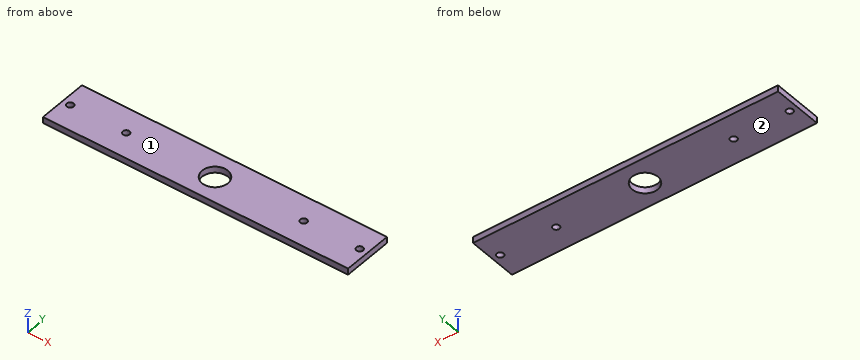
from build123d import *

# Parameters (mm, degrees)
SKETCH1_W               = 311.15
SKETCH1_H               = 50.8
BOSS_EXTRUDE1_DEPTH     = 6.35
F_1_CLEARANCE_HOLE1_D   = 26.19248
F_1_4_CLEARANCE_HOLE1_D = 6.7564


with BuildPart() as part:
    # Sketch1 → Boss-Extrude1 (new body)
    with BuildSketch(Plane.XY):
        Rectangle(SKETCH1_W, SKETCH1_H)
    extrude(amount=BOSS_EXTRUDE1_DEPTH)

    # 1 Clearance Hole1 (through all)
    with Locations(Plane.XY.offset(6.35)):
        with Locations((0, 0)):
            Hole(F_1_CLEARANCE_HOLE1_D / 2)

    # 1/4 Clearance Hole1 (through all)
    with Locations(Plane.XY.offset(6.35)):
        with Locations((-147.6375, 0), (-90.4875, 0)):
            f_1_4_clearance_hole1 = Hole(F_1_4_CLEARANCE_HOLE1_D / 2)

    # Mirror1: 1/4 Clearance Hole1 across plane
    add(f_1_4_clearance_hole1.mirror(Plane(origin=(0, 0, 0), x_dir=(0, 0, 1), z_dir=(1, 0, 0))), mode=Mode.SUBTRACT)


solid = part.part
Geometry: final body of the model. Coordinates: model frame, mm. Face numbers are marked on the shaded views. Round coordinates to 2 decimals unless told otherwise and drop trailing zeros. Order: outer loops, then holes, each group sorted by start corner. A loop starts at its lowest first (then second) coordinate and runs counter-clockwise, first axis right, second up. Notation, with made-up numbers: (3.5, -7.5) -> (48.5, -7.5) arc R8 ccw to (48.5, -0.5) -> close; hole circle Ø11 at (41, 7.25). An arc over 180 degrees is marked (long way). Put each result on its own line as item: value. Start each with the question number.
Q1. Line query: probe 1 along Y at (x, z) = (-89, 5.5); probe 2 along X at (y, z) = (4, 5.5) (3 decimals); probe 3 along Y at (x, z) = (-11, 2.75). Output: solid intervals per line, ascending.
Q2. Pull-direction query (Z, two-part tool) for the marked faces 1 and 2; classes: +Z half, -Z half, draft (parallel to the pull), parting line (faces both ways), or undercut.
Q3. Section C-C on z = 4. Return the cut outline in (x, y) (1 decimal).
Q4. Section B-B on y = 0. Return the cut outline in (x, z) (3 decimals), and give its area (3 significant figures).
Q5. Section A-A on x = 0. Return the cut outline in (y, z).
Q6. First-contact query: pin 1 (6 mm diameter, centred on x = -90.49, y = 0, fed in from +Z). Flat tip, straight axial feed; report the tip coordinate or a pass-through.
Ans:
1. probe 1: y = -25.4 to -3.03, 3.03 to 25.4
1. probe 2: x = -155.575 to -12.47, 12.47 to 155.575
1. probe 3: y = -25.4 to -7.11, 7.11 to 25.4
2. face 1: +Z half
2. face 2: -Z half
3. outline: (-155.6, -25.4) -> (155.6, -25.4) -> (155.6, 25.4) -> (-155.6, 25.4) -> close; hole circle Ø6.8 at (-147.6, 0); hole circle Ø6.8 at (-90.5, 0); hole circle Ø26.2 at (0, 0); hole circle Ø6.8 at (90.5, 0); hole circle Ø6.8 at (147.6, 0)
4. outline: (-155.575, 0) -> (-151.016, 0) -> (-151.016, 6.35) -> (-155.575, 6.35) -> close; (-144.259, 0) -> (-93.866, 0) -> (-93.866, 6.35) -> (-144.259, 6.35) -> close; (-87.109, 0) -> (-13.096, 0) -> (-13.096, 6.35) -> (-87.109, 6.35) -> close; (13.096, 0) -> (87.109, 0) -> (87.109, 6.35) -> (13.096, 6.35) -> close; (93.866, 0) -> (144.259, 0) -> (144.259, 6.35) -> (93.866, 6.35) -> close; (151.016, 0) -> (155.575, 0) -> (155.575, 6.35) -> (151.016, 6.35) -> close
4. area: 1,640 mm2
5. outline: (-25.4, 0) -> (-13.1, 0) -> (-13.1, 6.35) -> (-25.4, 6.35) -> close; (13.1, 0) -> (25.4, 0) -> (25.4, 6.35) -> (13.1, 6.35) -> close
6. pin 1: passes through
